Geometry: final body of the model. Coordinates: model frame, mm. Face numbers are marked on the shaded views. A direction names the side the tool comes from. Coordinates: 2 decimals unless noted, no trailing zeros. Order: outer loops, then holes, each group sorted by start corner. A loop starts at its lowest first (then second) coordinate and runs counter-clockwise, first axis right, second up. Notation, with made-up numbers: (59.25, -18) -> (116.25, -18) arc R35 ccw to (116.25, 15) -> close; hole circle Ø10 at (-16.5, -13). An arc over 180 degrees is marked (long way). Answer in a Markdown table with one row per item. Add a question column.
1) Section query D-D on y = 1. Return the cut outline in (x, z), then the cut area to 3 significant figures.
2) Contact query for flat-ended pins moving along their axis: P1, Ø2, axis at x = 11, z = 2.5, coming from the +Y side; P2, Ø4.5, axis at x = 22.03, z = 0, coming from the -Y side; P3, Ø4, axis at x = -0.5, z = 2.5, coming from the +Y side; P4, Ø2.5, axis at x = -12.5, y = 3.5, coming from the +Z side. Output: stop coordinate, or through.
3) Section query B-B on x = 23. Return the cut outline in (y, z).
4) Pull-direction query (Z, two-part tool) for the marked faces 5, 6, 7 and 8; classes: +Z half, -Z half, draft (parallel to the pull), parting line (faces both ways), or undercut.
5) Section query A-A on y = 5.5. Return the cut outline in (x, z).
6) Set-up query: the marked faces 1, 2, 3 and 4. Return all of +Z, -Z, +X, -X, +Y, -Y with unobstructed straight access to the full face (end or side cutting, diameter ignored); none if empty.
7) Ray query, line 1 (Y direction, x = 23, z = 5.25); line 2 (Z direction, x = 22.5, y = 4.25); line 3 (X direction, y = 8, z = 1.5). Return the intervals inside material, ascending. Write a range as from..to.
8) Section query C-C on x = -1. Return the cut outline in (y, z), then the cut area to 3 significant figures.
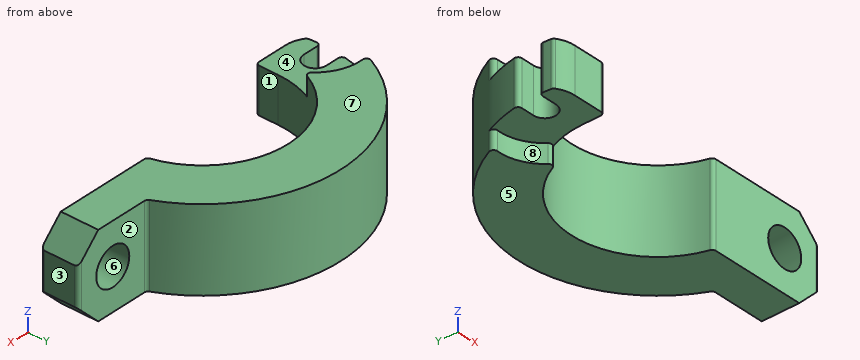
```python
from build123d import *

# Parameters (mm, degrees)
F1_DEPTH = 5.5
F3_DEPTH = 2.5
F5_R     = 2.5
F6_DEPTH = 5
F7_SIZE  = 3
F8_R     = 0.5


# Not quite as in the source:
# - a feature names something its author has since deleted; it is built from what else it names


with BuildPart() as f1:
    # F0 (on Top) → F1 (new body)
    with BuildSketch(Plane.XY):
        with BuildLine():
            ThreePointArc((-11.5, 0), (-1.2575412829, 11.4310362576), (11.2249721603, 2.5))
            Line((11.2249721603, 2.5), (27.2249721603, 2.5))
            Line((27.2249721603, 2.5), (27.2249721603, 7.5))
            Line((27.2249721603, 7.5), (16.9115345253, 7.5))
            ThreePointArc((16.9115345253, 7.5), (-2.5986969504, 18.3165710263), (-18.3303027798, 2.5))
            Line((-18.3303027798, 2.5), (-15.9687194227, 2.5))
            ThreePointArc((-15.9687194227, 2.5), (-14.4687194227, 1), (-15.9687194227, -0.5))
            Line((-15.9687194227, -0.5), (-18.4932420089, -0.5))
            ThreePointArc((-18.4932420089, -0.5), (-18.4505725724, -1.3514332211), (-18.3687238121, -2.1999967079))
            ThreePointArc((-18.3687238121, -2.1999967079), (-17.2336330893, -2.7947323247), (-15.9687194227, -3))
            Line((-15.9687194227, -3), (-11.5, -3))
            Line((-11.5, -3), (-11.5, 0))
        make_face()
    extrude(amount=F1_DEPTH)

    # F2 (on face) → F3 (cut)
    with BuildSketch(Plane.XY.offset(5.5)):
        with BuildLine():
            Line((-15.9687194227, -3), (-11.5, -3))
            Line((-11.5, -3), (-11.5, 0))
            ThreePointArc((-11.5, 0), (-11.3184211539, 2.0355202239), (-10.7794186814, 4.0067608976))
            ThreePointArc((-10.7794186814, 4.0067608976), (-13.5146873094, 6.472401636), (-17.1751666268, 6.8748564597))
            ThreePointArc((-17.1751666268, 6.8748564597), (-17.8869905716, 4.7228771203), (-18.3303027798, 2.5))
            Line((-18.3303027798, 2.5), (-15.9687194227, 2.5))
            ThreePointArc((-15.9687194227, 2.5), (-14.4687194227, 1), (-15.9687194227, -0.5))
            Line((-15.9687194227, -0.5), (-18.4932420089, -0.5))
            ThreePointArc((-18.4932420089, -0.5), (-18.4505725724, -1.3514332211), (-18.3687238121, -2.1999967079))
            ThreePointArc((-18.3687238121, -2.1999967079), (-17.2336330893, -2.7947323247), (-15.9687194227, -3))
        make_face()
    extrude(amount=-F3_DEPTH, mode=Mode.SUBTRACT)

    # F4: F1 across plane


with BuildPart() as f1_1:
    add(f1.part)
    add(f1.part.mirror(Plane.XY))

    # F5 (on face) → F6 (cut, through all)
    with BuildSketch(Plane(origin=(0, 7.5, 0), x_dir=(-1, 0, 0), z_dir=(0, 1, 0))):
        with Locations((-22.0312805773, 0)):
            Circle(F5_R)
    extrude(amount=-F6_DEPTH, mode=Mode.SUBTRACT)

    # F7
    f7_edges = [f1_1.edges().sort_by_distance(p)[0] for p in [
        (27.224972, 5, 5.5),
        (27.224972, 5, -5.5),
    ]]
    chamfer(f7_edges, length=F7_SIZE)

    # F8
    f8_edges = [f1_1.edges().sort_by_distance(p)[0] for p in [
        (-11.5, -3, 0),
        (-10.779419, 4.006761, 4.25),
        (-10.779419, 4.006761, -4.25),
        (-17.175167, 6.874856, 4.25),
        (-17.175167, 6.874856, -4.25),
        (-18.368724, -2.199997, 0),
        (-18.493242, -0.5, 0),
        (-18.330303, 2.5, 0),
        (11.224972, 2.5, 0),
        (16.911535, 7.5, 0),
        (27.224972, 2.5, 0),
        (27.224972, 7.5, 0),
    ]]
    fillet(f8_edges, radius=F8_R)


solid = f1_1.part
```
Result:
| question | item | result |
|---|---|---|
| 1 | outline | (-14.47, -3) -> (-11.46, -3) -> (-11.46, 3) -> (-14.47, 3) -> close |
| 1 | area | 18.1 mm2 |
| 2 | P1 | y = 15.56 |
| 2 | P2 | through |
| 2 | P3 | y = 18.5 |
| 2 | P4 | z = 3 |
| 3 | outline | (2.5, -5.5) -> (7.5, -5.5) -> (7.5, -2.3) -> (2.5, -2.3) -> close; (2.5, 2.3) -> (7.5, 2.3) -> (7.5, 5.5) -> (2.5, 5.5) -> close |
| 4 | face 5 | -Z half |
| 4 | face 6 | undercut |
| 4 | face 7 | +Z half |
| 4 | face 8 | draft |
| 5 | outline | (-17.66, -3) -> (-12, -3) -> (-12, -5.5) -> (-10.1, -5.5) -> (-10.1, 5.5) -> (-12, 5.5) -> (-12, 3) -> (-17.66, 3) -> close; (10.1, -5.5) -> (24.22, -5.5) -> (27.22, -2.5) -> (27.22, 2.5) -> (24.22, 5.5) -> (10.1, 5.5) -> close; hole circle Ø5 at (22.03, 0) |
| 6 | face 1 | +Z, -Z, +X, -Y |
| 6 | face 2 | +Z, -Z, +X, +Y |
| 6 | face 3 | +Z, -Z, +X, +Y, -Y |
| 6 | face 4 | +Z, -X, -Y |
| 7 | line 1 | 2.5..7.5 |
| 7 | line 2 | -5.5..-2.46, 2.46..5.5 |
| 7 | line 3 | -16.68..-8.26, 8.26..16.68 |
| 8 | outline | (11.46, -5.5) -> (18.47, -5.5) -> (18.47, 5.5) -> (11.46, 5.5) -> close |
| 8 | area | 77.2 mm2 |
